```python
from build123d import *

# Parameters (mm, degrees)
SKETCH1_W            = 25.4
SKETCH1_H            = 12.7
BOSS_EXTRUDE1_DEPTH  = 3.175
SKETCH2_R            = 1.9812
BOSS_EXTRUDE2_DEPTH  = 1.1938
LPATTERN1_COUNT      = 4
LPATTERN1_PITCH      = 6.35
LPATTERN1_COUNT_DIR2 = 2
LPATTERN1_PITCH_DIR2 = 6.35
SHELL2_T             = -1.1938
SKETCH3_R            = 2.5019
SKETCH3_R_2          = 1.9812
BOSS_EXTRUDE3_DEPTH  = 1.9812
LPATTERN2_COUNT      = 3
LPATTERN2_PITCH      = 6.35


with BuildPart() as part:
    # Sketch1 → Boss-Extrude1 (new body)
    with BuildSketch(Plane(origin=(0, 0, 0), x_dir=(1, 0, 0), z_dir=(0, 1, 0))):
        Rectangle(SKETCH1_W, SKETCH1_H)
    extrude(amount=BOSS_EXTRUDE1_DEPTH)

    # Sketch2 → Boss-Extrude2 (add)
    with BuildSketch(Plane(origin=(0, 3.175, 0), x_dir=(1, 0, 0), z_dir=(0, 1, 0))):
        with Locations(Location((-9.525, 3.175, 0), (0, 0, 270))):
            Circle(SKETCH2_R)
    boss_extrude2 = extrude(amount=BOSS_EXTRUDE2_DEPTH)

    # LPattern1: Boss-Extrude2 4 × 2
    with Locations(*[(i * LPATTERN1_PITCH, 0, j * LPATTERN1_PITCH_DIR2) for i in range(LPATTERN1_COUNT) for j in range(LPATTERN1_COUNT_DIR2) if (i, j) != (0, 0)]):
        add(boss_extrude2)

    # Shell2
    shell2_openings = [part.faces().sort_by_distance(p)[0] for p in [
        (0, 0, 0),
    ]]
    offset(amount=SHELL2_T, openings=shell2_openings, kind=Kind.INTERSECTION)

    # Sketch3 → Boss-Extrude3 (add)
    with BuildSketch(Plane.XZ.offset(-1.9812)):
        with Locations(Location((6.35, 0, 0), (0, 0, 90))):
            Circle(SKETCH3_R)
        with Locations(Location((6.35, 0, 0), (0, 0, 90))):
            Circle(SKETCH3_R_2, mode=Mode.SUBTRACT)
    boss_extrude3 = extrude(amount=BOSS_EXTRUDE3_DEPTH)

    # LPattern2: Boss-Extrude3 ×3
    with Locations(*[(-i * LPATTERN2_PITCH, 0, 0) for i in range(1, LPATTERN2_COUNT)]):
        add(boss_extrude3)


solid = part.part
```
Geometry: final body of the model. Coordinates: model frame, mm. A direction names the side the tool comes from. Coordinates: 2 decimals unless noted, no trailing zeros. Order: outer loops, then holes, each group sorted by start corner. A loop starts at its lowest first (then second) coordinate and runs counter-clockwise, first axis right, second up. Notation, with made-up numbers: M 73.25,76 L 123.25,76 A10 ccw 123.25,94 Z; hole C 56,67 d9. An arc over 180 degrees is marked long. Answer in a Markdown table with one row per item. Add a question column.
Q1. Section query B-B on x = -6.35. Return the cut outline in (y, z) (3 decimals), and give its area (3 significant figures).
Q2. Mould query, pull axis Z, two halves, no side actions, for faces 4 (the cylindrical face through (1.97, 3.76, -4.75)), 5 (the flat face through (-9, 4.369, -3)). Classes: released by +Z, released by -Z, zero draft, split by the parting line, or undercut.
Q3. Contact query for flat-ended pins moving along their axis: P1, Ø0.8, axis at x = -3, z = -3, coming from the -Y side (3 decimals); P2, Ø1.8, axis at x = -3.175, z = -3.175, coming from the -Y side. Output: stop coordinate, or through.
Q4. Section query A-A on y = 0.85. Return the cut outline in (x, z).
Q5. Reachability of faces 1 (the flat face through (-3, 3.175, -3)), 2 (the cylindrical face through (-8.2, 3.8, 1.7)), 3 (the flat face through (3, 4.369, 3)) from +Z, -Z, +X, -X, +Y, -Y: full face, straight path, thin tool, end or side. Return the list, or none.
Q6. Section query D-D on y = 2.45. Count the separate pieces of the cut face and the enclosed holes in it, and give its area (3 significant figures).
Q7. Section query C-C on z = -4.5. Return the cut outline in (x, y) (3 decimals).
Q8. Line query: L1, parallel to Z at x = 3, y = 1.9; L2, parallel to Z at x = 3.25, y = 2.2; L3, parallel to Z at x = -0.25, y = 1.1. Output: solid intervals per line, ascending.
Completed:
| question | item | result |
|---|---|---|
| 1 | outline | M 0,-6.35 L 3.175,-6.35 L 3.175,6.35 L 0,6.35 L 0,5.156 L 1.981,5.156 L 1.981,2.502 L 0,2.502 L 0,1.981 L 1.981,1.981 L 1.981,-1.981 L 0,-1.981 L 0,-2.502 L 1.981,-2.502 L 1.981,-5.156 L 0,-5.156 Z |
| 1 | area | 22.0 mm2 |
| 2 | face 4 | undercut |
| 2 | face 5 | zero draft |
| 3 | P1 | stops at y = 3.175 |
| 3 | P2 | stops at y = 1.98 |
| 4 | outline | M -12.7,-6.35 L 12.7,-6.35 L 12.7,6.35 L -12.7,6.35 Z; C -6.35,0 d5; C 0,0 d5; C 6.35,0 d5; hole M -11.51,-5.16 L 11.51,-5.16 L 11.51,5.16 L -11.51,5.16 Z; hole C -6.35,0 d3.96; hole C 0,0 d3.96; hole C 6.35,0 d3.96 |
| 5 | face 1 | -Y |
| 5 | face 2 | +Y |
| 5 | face 3 | +Z, -Z, +X, -X, +Y |
| 6 | separate pieces | 1 |
| 6 | enclosed holes | 8 |
| 6 | area | 307 mm2 |
| 7 | outline | M -12.7,0 L -11.506,0 L -11.506,1.981 L 11.506,1.981 L 11.506,0 L 12.7,0 L 12.7,3.175 L 10.998,3.175 L 10.998,4.369 L 8.052,4.369 L 8.052,3.175 L 4.648,3.175 L 4.648,4.369 L 1.702,4.369 L 1.702,3.175 L -1.702,3.175 L -1.702,4.369 L -4.648,4.369 L -4.648,3.175 L -8.052,3.175 L -8.052,4.369 L -10.998,4.369 L -10.998,3.175 L -12.7,3.175 Z |
| 8 | L1 | z = -6.35 to -5.16, 5.16 to 6.35 |
| 8 | L2 | z = -6.35 to -3.96, -2.39 to 2.39, 3.96 to 6.35 |
| 8 | L3 | z = -6.35 to -5.16, -2.49 to -1.97, 1.97 to 2.49, 5.16 to 6.35 |
